Source: CAD feature listing. Evaluate the final solid. Frame: model axes, mm. A direction names the side the tool comes from. Round coordinates to 2 decimals unless told otherwise and drop trailing zeros. Write each loop counter-clockwise with the first axis right and the second up, starting at its lowest first coordinate (ties: lowest second). Pieces come first, ordered by that corner, then holes. Notation, with made-up numbers: M 21,33.25 L 38,33.25 A16 ccw 38,46.25 Z; hole C -20,-33 d9. An arc over 180 degrees is marked long. Use a Markdown table: item, result.
```python
from build123d import *

# Parameters (mm, degrees)
SKETCH1_R                 = 18
EXTRUDE1_DEPTH            = 15
SKETCH2_R                 = 24
EXTRUDE2_DEPTH            = 5
CHAMFER2_SIZE             = 4
CHAMFER2_SIZE2            = 2
CHAMFER2_OF_MIRROR2_SIZE2 = 4
CHAMFER2_OF_MIRROR2_SIZE  = 2
EXTRUDE3_DEPTH            = 40.395431207
EXTRUDE3_DEPTH_BACK       = 40.395431207
SKETCH3_R                 = 8
CHAMFER3_SIZE             = 1


with BuildPart() as part:
    # Sketch1 → Extrude1 (new, symmetric)
    with BuildSketch(Plane.XY):
        Circle(SKETCH1_R)
    extrude(amount=EXTRUDE1_DEPTH, both=True)

    # Sketch2 → Extrude2 (add)
    with BuildSketch(Plane.XY.offset(15)):
        Circle(SKETCH2_R)
    extrude2 = extrude(amount=EXTRUDE2_DEPTH)

    # Chamfer2
    chamfer2_edges = [part.edges().sort_by_distance(p)[0] for p in [
        (-24, 0, 15),
    ]]
    chamfer2_side = [part.faces().sort_by_distance(p)[0] for p in [
        (-23.32117749, 0, 15),
    ]]
    chamfer(chamfer2_edges, length=CHAMFER2_SIZE, length2=CHAMFER2_SIZE2, reference=chamfer2_side[0])

    # Mirror2: Extrude2 across plane
    add(extrude2.mirror(Plane.XY))

    # Chamfer2 of Mirror2
    chamfer2_of_mirror2_edges = [part.edges().sort_by_distance(p)[0] for p in [
        (-24, 0, -15),
    ]]
    chamfer(chamfer2_of_mirror2_edges, length=CHAMFER2_OF_MIRROR2_SIZE, length2=CHAMFER2_OF_MIRROR2_SIZE2)

    # Sketch3 → Extrude3 (cut, two sides: drawn at the far end of the back side and taken through both)
    with BuildSketch(Plane.XY.offset(-EXTRUDE3_DEPTH_BACK)):
        Circle(SKETCH3_R)
    extrude(amount=EXTRUDE3_DEPTH + EXTRUDE3_DEPTH_BACK, mode=Mode.SUBTRACT)

    # Chamfer3
    chamfer3_edges = [part.edges().sort_by_distance(p)[0] for p in [
        (-8, 0, -20),
        (-8, 0, 20),
    ]]
    chamfer(chamfer3_edges, length=CHAMFER3_SIZE)


solid = part.part
```
Q1. Reachability of faces 1 (the cylindrical face through (-23.977, 1.055, 18.479)), 2 (the flat face through (-18, 3, 15)) from +Z, -Z, +X, -X, +Y, -Y: full face, straight path, thin tool, end or side. Return the list, or none.
Results are:
| item | result |
|---|---|
| face 1 | +Z, -Z |
| face 2 | none |
Q2. First-contact query: pin 1 Ø3 at (y, z) = (-4, 1) entering from +X; pin 2 Ø1.5 at (x, z) = (2, -5.5) entering from +Y; pin 3 Ø3 at (x, z) = (16, -10) entering from +Y. Flat tips, straight axial feed; report the tip coordinate or a pass-through.
Results are:
| item | result |
|---|---|
| pin 1 | x = 17.83 |
| pin 2 | y = 17.96 |
| pin 3 | y = 10.67 |
Q3. Mould query, pull axis Z, two halves, no side actions, for faces 3 (the flat face through (10, 0, 20)), 4 (the flat face through (10, 0, -20)), 5 (the cylindrical face through (-23.977, 1.055, -18.479)), 6 (the flat face through (-18, 3, -15)). Classes: +Z half, -Z half, draft (parallel to the pull), parting line (faces both ways), or undercut.
Results are:
| item | result |
|---|---|
| face 3 | +Z half |
| face 4 | -Z half |
| face 5 | draft |
| face 6 | undercut |
Q4. Section A-A on x = 0. Return loops of the section in (y, z), plus the area to 3 significant figures.
Results are:
| item | result |
|---|---|
| outline | M -24,-20 L -9,-20 L -8,-19 L -8,19 L -9,20 L -24,20 L -24,17 L -20,15 L -18,15 L -18,-15 L -20,-15 L -24,-17 Z; M 8,-19 L 9,-20 L 24,-20 L 24,-17 L 20,-15 L 18,-15 L 18,15 L 20,15 L 24,17 L 24,20 L 9,20 L 8,19 Z |
| area | 902 mm^2 |
Q5. Section C-C on z = 1.5. Return loops of the section in (x, y), plus the area to 3 significant figures.
Results are:
| item | result |
|---|---|
| outline | C 0,0 d36; hole C 0,0 d16 |
| area | 817 mm^2 |
Q6. Line query: L1, parallel to Y at x = 0, z = -8; L2, parallel to Z at x = 9, y = 16.5; L3, parallel to X at y = -2, z = -7. Output: solid intervals per line, ascending.
Results are:
| item | result |
|---|---|
| L1 | -18 to -8, 8 to 18 |
| L2 | -20 to -15, 15 to 20 |
| L3 | -17.89 to -7.75, 7.75 to 17.89 |
